Geometry: final body of the model. Coordinates: model frame, mm. A direction names the side the tool comes from. Round coordinates to 2 decimals unless told otherwise and drop trailing zeros. Order: outer loops, then holes, each group sorted by start corner. A loop starts at its lowest first (then second) coordinate and runs counter-clockwise, first axis right, second up. Notation, with made-up numbers: M -15.5,-26 L 4.5,-26 A27 cw 4.5,-1 Z; hole C 24,55 d9. An arc over 180 degrees is marked long. Return JSON: item names as keys, results as strings. Group by question number.
Q1. Contact query for flat-ended pins moving along their axis: pin 1 (3 mm diameter, centred on x = 17.5, y = 9.5, fed in from +Z); pin 2 (9.5 mm diameter, centred on x = 0, z = -32, fed in from +Y); pin 3 (2 mm diameter, centred on x = -21.5, y = 12, fed in from -Z); pin 4 (6.5 mm diameter, centred on x = 0.5, y = 11, fed in from -Z). Output: stop coordinate, or through.
Q2. Cut plane D-D on z = 16.5. Count the separate pieces of the cut face and the enclosed holes in it, and give its area (3 significant figures).
Q3. Access query for faces 1 (the face through (-0.303, 6.633, -11.739)), 2 (the face through (0, 12, -25)), 3 (the face through (-8, 6, -26)). Directions: +Z, -Z, +X, -X, +Y, -Y. A direction counts if a zero-diameter tool reaches every point of the face in a straight line with its end or side. Return the directions, or none.
Q4. Cut plane C-C on z = -20. Output: boundary loops of the cut face in (x, y).
Q5. Ray query, probe 1 along Z at (x, y) = (0, 1.85); probe 2 along X at (y, z) = (8, -14.5); probe 3 along X at (y, z) = (4.25, -38.5). Return the intervals inside material, ascending.
Q6. Mould query, pull axis Y, two halves, no side actions, for faces 4 (the face through (-0.325, 5.465, -45.464)), 5 (the face through (0, 8, -21.879)), 6 (the face through (0, 8, -38)). Classes: released by +Y, released by -Y, zero draft, split by the parting line, or undercut.
Q7. Cut plane B-B on x = 0. Output: boundary loops of the cut face in (y, z).
Q8. Cut plane A-A on z = -44. Output: boundary loops of the cut face in (x, y).
Autodesk Inventor part; units mm, degrees
ref_plane "YZ Plane" through (0, 0, 0) normal (1, 0, 0) x (0, 1, 0)
ref_plane "XZ Plane" through (0, 0, 0) normal (0, 1, 0) x (-1, 0, 0)
ref_plane "XY Plane" through (0, 0, 0) normal (0, 0, 1) x (1, 0, 0)
sketch "Sketch1" plane through (0, 0, 0) normal (0, 1, 0) x (-1, 0, 0)
  line L0 (0, -50) -> (8, -50)
  line L1 (8, -50) -> (8, -10)
  line L2 (0, 0) -> (0, -50) construction
  line L3 (0, -50) -> (-8, -50)
  line L4 (-8, -50) -> (-8, -10)
  line L5 (8, -10) -> (40.4833, 13.3417)
  line L6 (40.4833, 13.3417) -> (34.6478, 21.4626)
  line L7 (34.6478, 21.4626) -> (2.1646, -1.8792)
  line L8 (2.1646, -1.8792) -> (0, -1.8792)
  line L9 (-8, -10) -> (-40.4833, 13.3417)
  line L10 (-40.4833, 13.3417) -> (-34.6478, 21.4626)
  line L11 (-34.6478, 21.4626) -> (-2.1646, -1.8792)
  line L12 (-2.1646, -1.8792) -> (0, -1.8792)
  point P0 (4, -50)
  dimension "d0" = 16
  dimension "d17" = 10
  dimension "d18" = 40
extrude "Extrusion1" add sketch "Sketch1" along normal blind 16
sketch "Sketch2" plane through (0, 16, 0) normal (0, 1, 0) x (1, 0, 0)
  line L0 (8, 50) -> (-8, 50)
  line L1 (-8, 50) -> (-8, 10)
  line L2 (8, 10) -> (8, 50)
  line L3 (8, 10) -> (8, 50)
  line L4 (-8, 50) -> (8, 50)
  line L5 (8, 50) -> (8, 25)
  line L6 (8, 25) -> (-8, 25)
  line L7 (-8, 25) -> (-8, 50)
  line L8 (-8, 10) -> (-40.4833, -13.3417)
  line L9 (-40.4833, -13.3417) -> (-34.6478, -21.4626)
  line L10 (-34.6478, -21.4626) -> (-2.1646, 1.8792)
  line L11 (-2.1646, 1.8792) -> (2.1646, 1.8792)
  line L12 (2.1646, 1.8792) -> (34.6478, -21.4626)
  line L13 (34.6478, -21.4626) -> (40.4833, -13.3417)
  line L14 (40.4833, -13.3417) -> (8, 10)
  point P0 (0, 0)
  dimension "d6" = 25
extrude "Extrusion2" cut sketch "Sketch2" against normal blind 8 contours L2 L6 L1 L0
sketch "Sketch3" plane through (0, 0, 0) normal (0, -1, 0) x (1, 0, 0)
  line L0 (8, -50) -> (-8, -50)
  line L1 (8, -10) -> (8, -50)
  line L2 (-8, -50) -> (-8, -10)
  circle A0 centre (0, -44) radius 1.5
  circle A1 centre (0, -32) radius 1.5
  line L3 (40.4833, 13.3417) -> (8, -10)
  line L4 (34.6478, 21.4626) -> (40.4833, 13.3417)
  line L5 (2.1646, -1.8792) -> (34.6478, 21.4626)
  line L6 (-2.1646, -1.8792) -> (2.1646, -1.8792)
  line L7 (-34.6478, 21.4626) -> (-2.1646, -1.8792)
  line L8 (-40.4833, 13.3417) -> (-34.6478, 21.4626)
  line L9 (-8, -10) -> (-40.4833, 13.3417)
  point P0 (0, 0)
  dimension "d9" = 3
  dimension "d10" = 6
  dimension "d11" = 12
extrude "Extrusion3" cut sketch "Sketch3" against normal through all contours A0 | A1
sketch "Sketch4" plane through (0, 0, 0) normal (0, -1, 0) x (1, 0, 0)
  circle A0 centre (0, -32) radius 1.5
  circle A1 centre (0, -44) radius 1.5
  line L0 (8, -50) -> (-8, -50)
  line L1 (8, -10) -> (8, -50)
  line L2 (-8, -50) -> (-8, -10)
  circle A2 centre (0, -44) radius 3
  circle A3 centre (0, -32) radius 1.5
  circle A4 centre (0, -32) radius 3
  line L3 (40.4833, 13.3417) -> (8, -10)
  line L4 (34.6478, 21.4626) -> (40.4833, 13.3417)
  line L5 (2.1646, -1.8792) -> (34.6478, 21.4626)
  line L6 (-2.1646, -1.8792) -> (2.1646, -1.8792)
  line L7 (-34.6478, 21.4626) -> (-2.1646, -1.8792)
  line L8 (-40.4833, 13.3417) -> (-34.6478, 21.4626)
  line L9 (-8, -10) -> (-40.4833, 13.3417)
  point P0 (0, 0)
  dimension "d14" = 6
extrude "Extrusion4" cut sketch "Sketch4" against normal blind 3 contours A2 | A4
sketch "Sketch5" plane through (-2.1646, 0, -1.8792) normal (0.5835436, 0, 0.8120818) x (0.8120818, 0, -0.5835436)
  line L0 (-40, 0) -> (0, 0)
  line L1 (0, 0) -> (0, 16)
  line L2 (-40, 16) -> (0, 16)
  line L3 (-40, 0) -> (-40, 16)
  line L4 (-40, 0) -> (-40, 16) construction
  line L5 (-40, 8) -> (0, 8) construction
  line L6 (0, 0) -> (0, 16) construction
  circle A0 centre (-36, 13.5) radius 1.4
  circle A1 centre (-36, 8) radius 1.4
  circle A2 centre (-36, 2.5) radius 1.4
  point P0 (0.6612, 0)
  dimension "d19" = 2.8
  dimension "d20" = 11
  dimension "d21" = 4
extrude "Extrusion5" cut sketch "Sketch5" against normal through all contours A0 | A1 | A2
sketch "Sketch7" plane through (-2.1646, 0, -1.8792) normal (0, 0, 1) x (1, 0, 0)
  line L0 (0, 0) -> (4.3291, 0)
  line L1 (4.3291, 0) -> (4.3291, 16)
  line L2 (0, 16) -> (4.3291, 16)
  line L3 (0, 0) -> (0, 16)
  line L4 (0, 0) -> (0, 16) construction
  line L5 (0, 8) -> (4.3291, 8) construction
  line L6 (0.6646, 8) -> (3.6646, 8)
  circle A0 centre (2.1646, 8) radius 1.4
  point P0 (2.1646, 0)
  dimension "d24" = 2.8
extrude "Extrusion6" cut sketch "Sketch7" against normal blind 20 contours A0 L6 | L6 A0
sketch "Sketch8" plane through (34.6478, 0, 21.4626) normal (-0.5835436, 0, 0.8120818) x (0.8120818, 0, 0.5835436)
  line L0 (-40, 0) -> (0, 0)
  line L1 (0, 0) -> (0, 16)
  line L2 (-40, 16) -> (0, 16)
  line L3 (-40, 0) -> (-40, 16)
  line L4 (0, 0) -> (0, 16) construction
  line L5 (0, 8) -> (-40, 8) construction
  line L6 (-40, 0) -> (-40, 16) construction
  circle A0 centre (-4, 8) radius 1.4
  circle A1 centre (-4, 3) radius 1.4
  circle A2 centre (-4, 13) radius 1.4
  point P0 (-40.6612, 0)
  dimension "d27" = 2.8
  dimension "d28" = 4
  dimension "d29" = 10
extrude "Extrusion7" cut sketch "Sketch8" against normal through all contours A0 | A1 | A2
properties part number "B1_head_Y"
Result sheet:
{
 "1": {"pin 1": "stops at z = 10.22", "pin 2": "stops at y = 8", "pin 3": "stops at z = -1.02", "pin 4": "stops at z = -50"},
 "2": {"separate pieces": "2", "enclosed holes": "6", "area": "290 mm²"},
 "3": {"face 1": "+Z", "face 2": "-Z, +X, -X, +Y", "face 3": "-Z, -X, +Y, -Y"},
 "4": {"outline": "M -8,0 L 8,0 L 8,16 L -8,16 Z; hole C 0,8 d2.8"},
 "5": {"probe 1": "z = -50 to -47, -41 to -35, -29 to -1.88", "probe 2": "x = -8 to -1.4, 1.4 to 8", "probe 3": "x = -8 to 8"},
 "6": {"face 4": "zero draft", "face 5": "undercut", "face 6": "released by +Y"},
 "7": {"outline": "M 0,-50 L 8,-50 L 8,-45.5 L 3,-45.5 L 3,-47 L 0,-47 Z; M 0,-41 L 3,-41 L 3,-42.5 L 8,-42.5 L 8,-33.5 L 3,-33.5 L 3,-35 L 0,-35 Z; M 0,-29 L 3,-29 L 3,-30.5 L 8,-30.5 L 8,-25 L 16,-25 L 16,-1.88 L 9.4,-1.88 L 9.4,-21.88 L 6.6,-21.88 L 6.6,-1.88 L 0,-1.88 Z"},
 "8": {"outline": "M -8,0 L -3,0 L -3,3 L -1.5,3 L -1.5,8 L -8,8 Z; M 1.5,3 L 3,3 L 3,0 L 8,0 L 8,8 L 1.5,8 Z"}
}
